from build123d import *

# Parameters (mm, degrees)
EXTRUS_O1_DEPTH = 5
FILETE1_R       = 0.1
FILETE2_R       = 0.2
FILETE3_R       = 0.03


with BuildPart() as part:
    # Esboço1 → Revolução1 (revolve)
    with BuildSketch(Plane.XY, mode=Mode.PRIVATE) as revolu_o1_sk:
        with BuildLine():
            Line((0, 2.232465991), (0, 2.675))
            Line((0, 2.675), (4, 2.675))
            Line((4, 2.675), (4, 2.775))
            Line((4, 2.775), (27.45, 2.825))
            Line((27.45, 2.825), (27.45, 3.325))
            Line((27.45, 3.325), (28.4, 3.325))
            Line((28.4, 3.325), (28.4, 3.65))
            Line((28.4, 3.65), (29.75, 3.531890304))
            Line((29.75, 3.531890304), (29.75, 3.225))
            Line((29.75, 3.225), (33.653170972, 3.254044116))
            ThreePointArc((33.653170972, 3.254044116), (33.761490772, 3.223126579), (33.83592072, 3.138573305))
            Line((33.83592072, 3.138573305), (34.6, 1.5))
            Line((34.6, 1.5), (34.6, 1.073205081))
            Line((34.6, 1.073205081), (34.3, 0.9))
            Line((34.3, 0.9), (34.3, 0.2))
            Line((34.3, 0.2), (34.517634594, 0.2))
            Line((34.517634594, 0.2), (34.517634594, 0))
            Line((34.517634594, 0), (33.7, 0))
            Line((33.7, 0), (33.7, 1.652085159))
            Line((33.7, 1.652085159), (3, 1.92))
            Line((3, 1.92), (3, 1.97))
            Line((3, 1.97), (0, 2.232465991))
        make_face()
    revolve(revolu_o1_sk.sketch.rotate(Axis((0, 0, 0), (1, 0, 0)), 90), axis=Axis((0, 0, 0), (1, 0, 0)))

    # Esboço2 → Extrusão1 (cut, symmetric)
    with BuildSketch(Plane.XY):
        with BuildLine():
            Line((0, 1), (0, -1))
            Line((0, -1), (2, -1))
            ThreePointArc((2, -1), (3, 0), (2, 1))
            Line((2, 1), (0, 1))
        make_face()
    extrude(amount=EXTRUS_O1_DEPTH, both=True, mode=Mode.SUBTRACT)

    # Filete1
    filete1_edges = [part.edges().sort_by_distance(p)[0] for p in [
        (33.7, 0, -1.652085159),
    ]]
    fillet(filete1_edges, radius=FILETE1_R)

    # Filete2
    filete2_edges = [part.edges().sort_by_distance(p)[0] for p in [
        (0, -1, -2.238512624),
        (0, -1, 2.238512624),
        (0, 1, -2.238512624),
        (0, 1, 2.238512624),
    ]]
    fillet(filete2_edges, radius=FILETE2_R)

    # Filete3
    filete3_edges = [part.edges().sort_by_distance(p)[0] for p in [
        (3, 0, -1.92),
    ]]
    fillet(filete3_edges, radius=FILETE3_R)


solid = part.part
CAD build for the part. Positions are in the model's coordinates, mm. A direction names the side the tool comes from. Give positions to 0.01 mm unless a question says otherwise; leave off trailing zeros. Write each loop counter-clockwise with the first axis right and the second up, starting at its lowest first coordinate (ties: lowest second). Pieces come first, ordered by that corner, then holes. Notation, with made-up numbers: M 84,54 L 143,54 A20 ccw 143,77 Z; hole C 7.5,66.25 d5. An arc over 180 degrees is marked long. Put each result on its own line as item: value. Start each with the question number.
(1) Which spindle directions (+Z, -Z, +X, -X, +Y, -Y) get a long thin tool onto all of the face, cutting with end or side? Do faces 4 (the face through (31.73, 1.97, -2.57)), 5 (the face through (3, 0, 2.2)), 6 (the face through (27.45, 3, 1)). Say none if no direction does.
(2) Probe L1, parallel to Y at x = 21.5, z = 1.5; L2, parallel to Y at x = 12, z = -1; L3, parallel to Z at x = 10, y = -0.75. List the from-to ranges inside material, lowest first.
(3) Band-saw the part on A-A, the plane x = 19. Write the cut outline in (y, z), and give its area (3 significant figures).
(4) Band-saw the part on B-B, the plane x = 26.5. Write the cut outline in (y, z), and give its area (3 significant figures).
(5) Mould opens along Z. For faces 1 (the face through (18.101, -0.537, 1.706)), 2 (the face through (0, -2.4, 0)), 3 (the face through (2.028, 2.373, 1.234)) say: +Z half, -Z half, draft (parallel to the pull), parting line (faces both ways), or undercut.
(6) Flat gauge pins, fed straight in: pin 1 Ø0.8 at (x, z) = (1, -2) entering from +Y; pin 2 Ø1 at (x, z) = (21, 1.5) entering from +Y; pin 3 Ø1 at (x, z) = (10.5, -2.5) entering from -Y. Where does each tip first touch, or does it go through?
Response values:
1. face 4: none
1. face 5: +Z, -Z, -X
1. face 6: -X
2. L1: y = -2.38 to -0.92, 0.92 to 2.38
2. L2: y = -2.61 to -1.55, 1.55 to 2.61
2. L3: z = -2.69 to -1.7, 1.7 to 2.69
3. outline: C 0,0 d5.61; hole C 0,0 d3.56
3. area: 14.8 mm2
4. outline: C 0,0 d5.65; hole C 0,0 d3.43
4. area: 15.8 mm2
5. face 1: undercut
5. face 2: draft
5. face 3: parting line
6. pin 1: stops at y = 2.14
6. pin 2: stops at y = 2.63
6. pin 3: stops at y = -1.94
